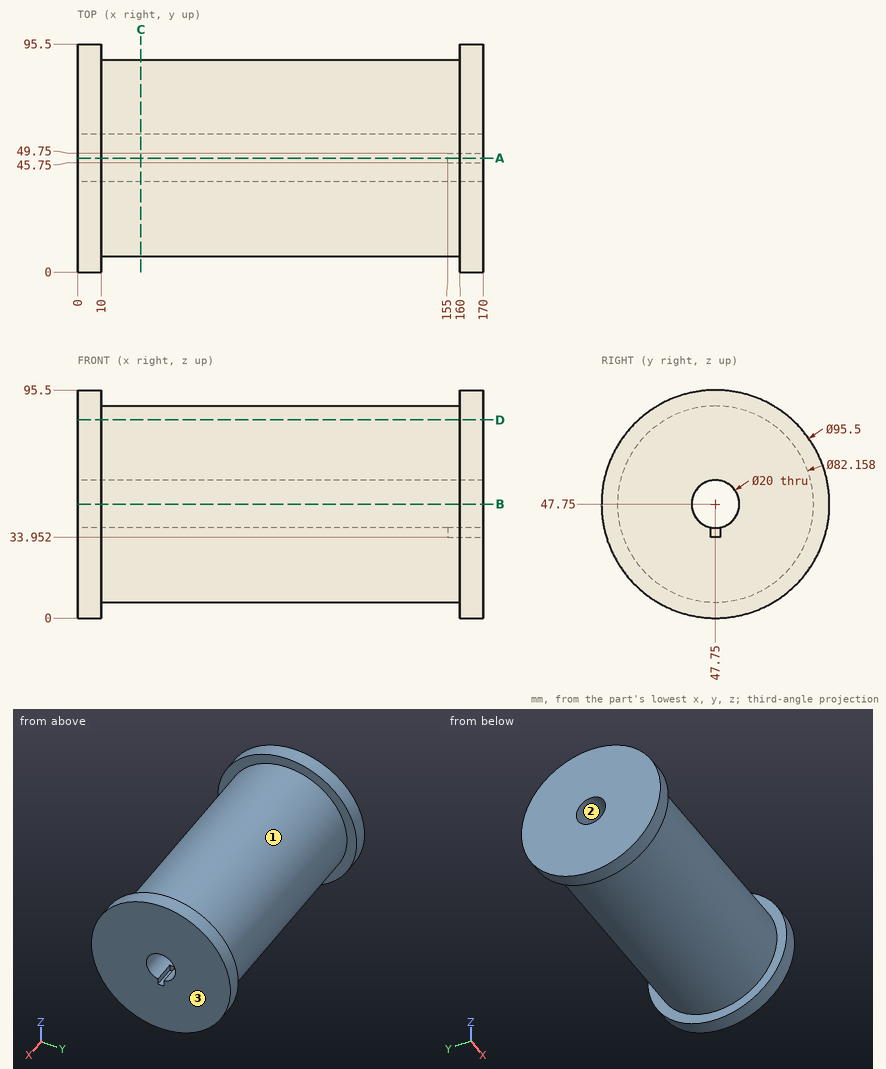
Can you work these out from the drawing? Everything is in mm from the part's minimum corner. Coordinates: 2 decimals unless noted, no trailing zeros. Loops run counter-clockwise (first coordinate to the right, second up) from the corner with the lowest first, then second, coordinate; pieces in that order, holes last. Notation, with made-up numbers: (-4, 37.25) - (29, 37.25) arc R22 cw to (29, 54.25) - close; hole circle Ø5 at (17, 14). An arc over 180 degrees is marked (long way). Put each result on its own line as item: value. Start each with the question number.
Item 1: Suppose I cut it at C-C (x = 26.5). Please give me the cut outline in (y, z), and give its area (3 significant figures).
Item 2: If we mould it in two halves opening along Y, with no side actions, what happens to the marked faces 1, 2 and 3? For each: +Y half, -Y half, draft (parallel to the pull), parting line (faces both ways), or undercut.
Item 3: If I drill on line 1 along Y through (x, z) = (130, 47); line 2 along X through (y, z) = (5.5, 29.5); line 3 along Y through (x, z) = (11, 55), over which ranges is the centre line in solid material (lowest first)?
Item 4: Suppose I cut it at B-B (z = 47.75). Please give me the cut outline in (x, y).
Item 5: Suppose I cut it at D-D (z = 83). Please give me the cut outline in (x, y).
Item 6: Suppose I cut it at A-A (y = 47.75). Please give me the cut outline in (x, z), and give its area (3 significant figures).
Item 7: For pin 1 (12 mm diameter, centred on x = 89, y = 36.5, fed in from +Z); pin 2 (3 mm diameter, centred on y = 21.5, z = 79.5, fed in from -X); pin 3 (1.2 mm diameter, centred on x = 165, z = 36.5, fed in from -Y); pin 4 (1.5 mm diameter, centred on x = 85.5, z = 50, fed in from +Y), each with a flat end and sliding along its axis, tell me the tip position at first contact or that it passes through.
Here are the results:
1. outline: circle Ø82.16 at (47.75, 47.75); hole circle Ø20 at (47.75, 47.75)
1. area: 4,990 mm²
2. face 1: parting line
2. face 2: undercut
2. face 3: draft
3. line 1: 6.68 to 37.78, 57.72 to 88.82
3. line 2: 0 to 10, 160 to 170
3. line 3: 7.32 to 40.86, 54.64 to 88.18
4. outline: (0, 0) - (10, 0) - (10, 6.67) - (160, 6.67) - (160, 0) - (170, 0) - (170, 37.75) - (0, 37.75) - close; (0, 57.75) - (170, 57.75) - (170, 95.5) - (160, 95.5) - (160, 88.83) - (10, 88.83) - (10, 95.5) - (0, 95.5) - close
5. outline: (0, 15.54) - (10, 15.54) - (10, 26.66) - (160, 26.66) - (160, 15.54) - (170, 15.54) - (170, 79.96) - (160, 79.96) - (160, 68.84) - (10, 68.84) - (10, 79.96) - (0, 79.96) - close
6. outline: (0, 0) - (10, 0) - (10, 6.67) - (160, 6.67) - (160, 0) - (170, 0) - (170, 33.95) - (155, 33.95) - (155, 37.75) - (0, 37.75) - close; (0, 57.75) - (170, 57.75) - (170, 95.5) - (160, 95.5) - (160, 88.83) - (10, 88.83) - (10, 95.5) - (0, 95.5) - close
6. area: 10,800 mm²
7. pin 1: z = 88.49
7. pin 2: x = 0
7. pin 3: y = 1.2
7. pin 4: y = 88.8
